```python
from build123d import *

# Parameters (mm, degrees)
SKETCH1_W           = 300
SKETCH1_H           = 22.32
BOSS_EXTRUDE1_DEPTH = 5
SKETCH2_W           = 5
SKETCH2_H           = 20
BOSS_EXTRUDE2_DEPTH = 5
SKETCH3_W           = 5
SKETCH3_H           = 20
BOSS_EXTRUDE3_DEPTH = 5
SKETCH4_W           = 10
SKETCH4_H           = 10
CUT_EXTRUDE1_DEPTH  = 5


with BuildPart() as part:
    # Sketch1 → Boss-Extrude1 (new body)
    with BuildSketch(Plane(origin=(0, 0, 0), x_dir=(0, 0, -1), z_dir=(1, 0, 0))):
        with Locations((150, 11.16)):
            Rectangle(SKETCH1_W, SKETCH1_H)
    extrude(amount=BOSS_EXTRUDE1_DEPTH)

    # Sketch2 → Boss-Extrude2 (add)
    with BuildSketch(Plane(origin=(0, 22.32, 0), x_dir=(1, 0, 0), z_dir=(0, 1, 0))):
        with Locations((2.5, 30)):
            Rectangle(SKETCH2_W, SKETCH2_H)
        with Locations((2.5, 270)):
            Rectangle(SKETCH2_W, SKETCH2_H)
        with Locations((2.5, 150)):
            Rectangle(SKETCH2_W, SKETCH2_H)
    extrude(amount=BOSS_EXTRUDE2_DEPTH)

    # Sketch3 → Boss-Extrude3 (add)
    with BuildSketch(Plane.XZ):
        with Locations((2.5, -30)):
            Rectangle(SKETCH3_W, SKETCH3_H)
        with Locations((2.5, -150)):
            Rectangle(SKETCH3_W, SKETCH3_H)
        with Locations((2.5, -270)):
            Rectangle(SKETCH3_W, SKETCH3_H)
    extrude(amount=BOSS_EXTRUDE3_DEPTH)

    # Sketch4 → Cut-Extrude1 (cut)
    with BuildSketch(Plane(origin=(5, 0, 0), x_dir=(0, 0, -1), z_dir=(1, 0, 0))):
        with Locations((210, 11)):
            Rectangle(SKETCH4_W, SKETCH4_H)
    extrude(amount=-CUT_EXTRUDE1_DEPTH, mode=Mode.SUBTRACT)


solid = part.part
```
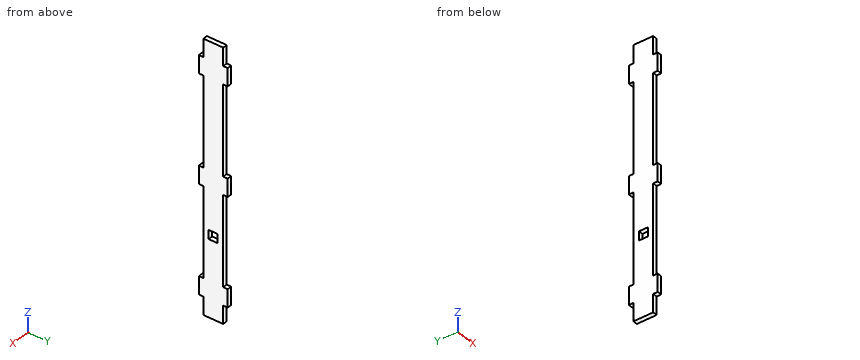
Read the model definition and answer for the solid it produces. Units are mm, in the model's axes. Round coordinates to 2 decimals unless told otherwise and drop trailing zeros. Write each loop counter-clockwise with the first axis right and the second up, starting at its lowest first coordinate (ties: lowest second). Pieces come first, ordered by that corner, then holes. Notation, with made-up numbers: M -24.5,-10 L -19.5,-10 A14 cw -19.5,14 Z; hole C 58,-35 d6. An arc over 180 degrees is marked long. One line per item, written item: value.
Q1. Find section A-A on z = -208. Write down the section's boundary in (x, y), plus the area to 3 significant figures.
Data:
outline: M 0,0 L 5,0 L 5,6 L 0,6 Z; M 0,16 L 5,16 L 5,22.32 L 0,22.32 Z
area: 61.6 mm2
Q2. Find section D-D on z = -85. Write down the section's boundary in (x, y), plus the area to 3 significant figures.
Data:
outline: M 0,0 L 5,0 L 5,22.32 L 0,22.32 Z
area: 112 mm2
Q3. Straight lines are drawn through the part: line 1 (Z direction, x = 2.25, y = 8.5); line 2 (Y direction, x = 3.1, z = -17). For each, find the intervals that lie inside material, in ascending order. Write a range as [from, to].
Data:
line 1: [-300, -215], [-205, 0]
line 2: [0, 22.32]
Q4. Flat-ended cylindrical pins translate along their axes: pin 1 Ø2.5 at (x, z) = (3, -288) entering from -Y; pin 2 Ø2.5 at (x, z) = (3.5, -12.5) entering from +Y. Find the tip coordinate at first contact, or state that the pin passes through.
Data:
pin 1: y = 0
pin 2: y = 22.32
Q5. Find section B-B on y = 12.5. Write down the section's boundary in (x, z), plus the area to 3 significant figures.
Data:
outline: M 0,-300 L 5,-300 L 5,-215 L 0,-215 Z; M 0,-205 L 5,-205 L 5,0 L 0,0 Z
area: 1,450 mm2
